For this review, take the finished solid that the model builds, in its own axes (mm). A direction names the side the tool comes from. Give positions to 0.01 mm unless a question says otherwise; leave off trailing zeros. Loops run counter-clockwise (first coordinate to the right, second up) from the corner with the lowest first, then second, coordinate; pieces in that order, holes last.
```python
from build123d import *

# Parameters (mm, degrees)
F1_DEPTH = 20
F2_R     = 1
F3_R     = 2
F4_R     = 3


with BuildPart() as f1:
    # F0 (on Top) → F1 (new body)
    with BuildSketch(Plane.XY):
        Polygon((0, -4.999999), (0, 0), (-86, 0), (-86, 48), (-79, 48), (-79, 52.999999), (-90.999999, 52.999999), (-90.999999, -4.999999), align=None)
        Polygon((0, 51.528051), (0, 0), (0, -4.999999), (5, -4.999999), (5, 0), (5, 51.528051), align=None)
    extrude(amount=F1_DEPTH)

    # F2
    f2_edges = [f1.edges().sort_by_distance(p)[0] for p in [
        (0, 0, 10),
    ]]
    fillet(f2_edges, radius=F2_R)

    # F3
    f3_edges = [f1.edges().sort_by_distance(p)[0] for p in [
        (-86, 48, 10),
        (-86, 0, 10),
    ]]
    fillet(f3_edges, radius=F3_R)

    # F4
    f4_edges = [f1.edges().sort_by_distance(p)[0] for p in [
        (5, 23.264026, 0),
        (5, 51.528051, 10),
        (5, 23.264026, 20),
    ]]
    fillet(f4_edges, radius=F4_R)


solid = f1.part
```
Item 1: Take a section at B-B on x = -82. Give the boundary of the cut face in (y, z).
Answer:
outline: (-5, 0) - (0, 0) - (0, 20) - (-5, 20) - close; (48, 0) - (53, 0) - (53, 20) - (48, 20) - close
Item 2: The part is to be moulded in two halves that separate along X. For faces 5 (the flat face through (-86, 24, 10)), 6 (the flat face through (-44, -5, 10)), 7 (the cylindrical face through (4.1, 50.67, 10.14)), say which applies: released by +X, released by -X, zero draft, split by the parting line, or undercut.
Answer:
face 5: undercut
face 6: zero draft
face 7: released by +X
Item 3: Clearance check with flat-ended pins moving along their axes: pin 1 Ø10 at (x, z) = (-53, 11.5) entering from +Y; pin 2 Ø8 at (x, y) = (-81, 34) entering from +Z; pin 3 Ø1.6 at (x, z) = (1.5, 11.5) entering from +Y. State where each tip first meets the part, or that it passes through.
Answer:
pin 1: stops at y = 0
pin 2: passes through
pin 3: stops at y = 51.53
Item 4: Tool access review of faces 1 (the cylindrical face through (-85.43, 47.4, 10.14)), 2 (the flat face through (1, 51.528, 10)), 3 (the flat face through (-79, 50, 10)), 4 (the flat face through (-85, 53, 10)): name each direction out of +Z, -Z, +X, -X, +Y, -Y from which nothing blocks a thin tool from reaching the whole face with its end or side.
Answer:
face 1: +Z, -Z
face 2: +Z, -Z, +X, +Y
face 3: +Z, -Z, +Y
face 4: +Z, -Z, +X, -X, +Y
Item 5: Take a section at A-A on y = 32. Give the boundary of the cut face in (x, z), and give its area (3 significant figures).
Answer:
outline: (-91, 0) - (-86, 0) - (-86, 20) - (-91, 20) - close; (0, 0) - (2, 0) arc R3 ccw to (5, 3) - (5, 17) arc R3 ccw to (2, 20) - (0, 20) - close
area: 196 mm2
Item 6: For L1, parallel to X at y = 19.5, z = 14; L2, parallel to Y at x = -73.5, z = 8.75; L3, parallel to X at y = 21, z = 18.5, list the stretches that pass through material, from the lowest coordinate up.
Answer:
L1: x = -91 to -86, 0 to 5
L2: y = -5 to 0
L3: x = -91 to -86, 0 to 4.6
Item 7: Take a section at C-C on z = 5.5. Give the boundary of the cut face in (x, y), and give its area (3 significant figures).
Answer:
outline: (-91, -5) - (5, -5) - (5, 48.53) arc R3 ccw to (2, 51.53) - (0, 51.53) - (0, 1) arc R1 cw to (-1, 0) - (-84, 0) arc R2 cw to (-86, 2) - (-86, 46) arc R2 cw to (-84, 48) - (-79, 48) - (-79, 53) - (-91, 53) - close
area: 1,040 mm2
